Could you check a few things on this model? Use its own coordinates, in mm. Face numbers are marked on the shaded views. A direction names the side the tool comes from. Round coordinates to 2 decimals unless told otherwise and drop trailing zeros. Loops run counter-clockwise (first coordinate to the right, second up) from the corner with the lowest first, then second, coordinate; pieces in that order, holes last. Notation, with made-up numbers: (-7.75, 82) - (41.25, 82) arc R11 ccw to (41.25, 91) - close; hole circle Ø10 at (6, -34.5). An arc over 180 degrees is marked (long way). Put each result on its own line as item: value. Start each with the question number.
from build123d import *

# Parameters (mm, degrees)
F0_W     = 15.875
F0_H     = 14.35001
F0_R     = 2.15265
F1_DEPTH = 1.5875
F2_W     = 15.875
F2_H     = 14.35001
F2_R     = 4
F3_DEPTH = 6.35
F4_SIZE  = 0.254
F5_W     = 3.175
F5_H     = 14.35001
F6_DEPTH = 1.5875


with BuildPart() as f1:
    # F0 (on Top) → F1 (new body)
    with BuildSketch(Plane.XY):
        Rectangle(F0_W, F0_H)
        Circle(F0_R, mode=Mode.SUBTRACT)
    extrude(amount=F1_DEPTH)

    # F2 (on face) → F3 (join)
    with BuildSketch(Plane.XY.offset(1.5875)):
        Rectangle(F2_W, F2_H)
        Circle(F2_R, mode=Mode.SUBTRACT)
    extrude(amount=F3_DEPTH)

    # F4
    f4_edges = [f1.edges().sort_by_distance(p)[0] for p in [
        (-4, 0, 7.9375),
    ]]
    chamfer(f4_edges, length=F4_SIZE)

    # F5 (on face) → F6 (join)
    with BuildSketch(Plane(origin=(0, 0, 0), x_dir=(1, 0, 0), z_dir=(0, 0, -1))):
        with Locations((-6.35, 0)):
            Rectangle(F5_W, F5_H)
        with Locations((6.35, 0)):
            Rectangle(F5_W, F5_H)
    extrude(amount=F6_DEPTH)


solid = f1.part
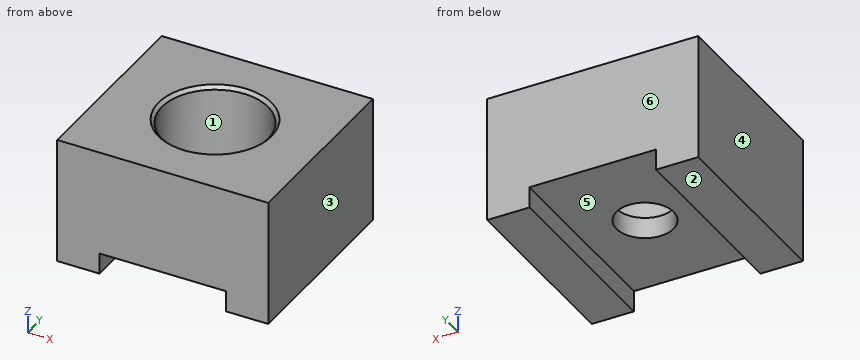
Item 1: Suppose I cut it at B-B, the plane z = 0.75. List the corners of the cut face in (x, y) for me (1 decimal), then the cut area to 3 significant figures.
Item 2: Will these pins go through, and if not, where does the flat tip stop? P1, Ø4, axis at x = 0, y = 1, coming from the -Z side; P2, Ø2.5, axis at x = -0.5, y = -0.5, coming from the +Z side.
Item 3: Suppose I cut it at A-A, the plane y = 0. List the corners of the cut face in (x, z) for me.
Item 4: I need wall thicknesses on line 1 (Y direction, x = 0, z = 4) (3 decimals); line 2 (Y direction, x = 0, z = 0.45) (3 decimals); line 3 (Z direction, x = -4.5, y = -6.25). Which ranges of each line are inside material? Lowest first, please. Write a range as from..to.
Item 5: On a 3-axis mill with a long thin cutter (end or side, diameter ignored), from which of +Z, -Z, +X, -X, +Y, -Y can I reach the whole of each face in a straight line? I mean the marked faces 5 and 6. Say none if no direction works.
Item 6: Thinking about a two-plate mould opening in X: for the marked faces 1, 2, 3 and 4, which applies, released by +X, released by -X, zero draft, split by the parting line, or undercut?
Item 7: Suppose I cut it at D-D, the plane y = -5. List the corners of the cut face in (x, z) for me.
Numbers:
1. outline: (-7.9, -7.2) - (7.9, -7.2) - (7.9, 7.2) - (-7.9, 7.2) - close; hole circle Ø4.3 at (0, 0)
1. area: 213 mm^2
2. P1: z = 0
2. P2: through
3. outline: (-7.94, -1.59) - (-4.76, -1.59) - (-4.76, 0) - (-2.15, 0) - (-2.15, 1.59) - (-4, 1.59) - (-4, 7.68) - (-4.25, 7.94) - (-7.94, 7.94) - close; (2.15, 0) - (4.76, 0) - (4.76, -1.59) - (7.94, -1.59) - (7.94, 7.94) - (4.25, 7.94) - (4, 7.68) - (4, 1.59) - (2.15, 1.59) - close
4. line 1: -7.175..-4, 4..7.175
4. line 2: -7.175..-2.153, 2.153..7.175
4. line 3: 0..7.94
5. face 5: -Z, +Y, -Y
5. face 6: +Z, -Z, +X, -X, +Y
6. face 1: undercut
6. face 2: zero draft
6. face 3: released by +X
6. face 4: released by -X
7. outline: (-7.94, -1.59) - (-4.76, -1.59) - (-4.76, 0) - (4.76, 0) - (4.76, -1.59) - (7.94, -1.59) - (7.94, 7.94) - (-7.94, 7.94) - close
